Here's how the part is built. I have some questions about the finished solid (model axes, mm). A direction names the side the tool comes from. Round coordinates to 2 decimals unless told otherwise and drop trailing zeros. Order: outer loops, then holes, each group sorted by start corner. A loop starts at its lowest first (then second) coordinate and runs counter-clockwise, first axis right, second up. Notation, with made-up numbers: (-22.75, 37.5) -> (2.25, 37.5) arc R10 cw to (2.25, 53.5) -> close; hole circle Ø11 at (26.5, 42.25). An arc over 180 degrees is marked (long way). One line per item, written item: value.
```python
from build123d import *

# Parameters (mm, degrees)
SKICA1_W                 = 60
SKICA1_H                 = 100
P_IDAT_VYSUNUT_M1_DEPTH  = 30
SKICA2_W                 = 60
SKICA2_H                 = 30
P_IDAT_VYSUNUT_M2_DEPTH  = 80
SKICA3_R                 = 12.5
ODEBRAT_VYSUNUT_M1_DEPTH = 80
ZAOBLIT2_R               = 10
ZKOSEN_1_SIZE            = 5


with BuildPart() as part:
    # Skica1 → Přidat vysunutím1 (new body)
    with BuildSketch(Plane.XY):
        with Locations((30, 50)):
            Rectangle(SKICA1_W, SKICA1_H)
    extrude(amount=P_IDAT_VYSUNUT_M1_DEPTH)

    # Skica2 → Přidat vysunutím2 (add)
    with BuildSketch(Plane(origin=(0, 0, 0), x_dir=(-1, 0, 0), z_dir=(0, 0, -1))):
        with Locations((-30, 85)):
            Rectangle(SKICA2_W, SKICA2_H)
    extrude(amount=P_IDAT_VYSUNUT_M2_DEPTH)

    # Skica3 → Odebrat vysunutím1 (cut)
    with BuildSketch(Plane(origin=(0, 0, 0), x_dir=(-1, 0, 0), z_dir=(0, 0, -1))):
        with Locations((-30, 40)):
            Circle(SKICA3_R)
    extrude(amount=-ODEBRAT_VYSUNUT_M1_DEPTH, mode=Mode.SUBTRACT)

    # Zaoblit2
    zaoblit2_edges = [part.edges().sort_by_distance(p)[0] for p in [
        (30, 70, 0),
    ]]
    fillet(zaoblit2_edges, radius=ZAOBLIT2_R)

    # Zkosení1
    zkosen_1_edges = [part.edges().sort_by_distance(p)[0] for p in [
        (60, 0, 15),
        (0, 0, 15),
    ]]
    chamfer(zkosen_1_edges, length=ZKOSEN_1_SIZE)


solid = part.part
```
Q1. I need wall thicknesses on line 1 along Y through (x, z) = (30, 10.5); line 2 along Y through (x, z) = (7.5, -63.5); line 3 along Y through (x, z) = (34.5, 9). Which ranges of each line are inside material? Lowest first, please.
Answers:
line 1: 0 to 27.5, 52.5 to 100
line 2: 70 to 100
line 3: 0 to 28.34, 51.66 to 100
Q2. Which directions (+Z, -Z, +X, -X, +Y, -Y) give clear straight access to the entire face, cutting with the end or side of a thin tool? Please do faces 4 (the face through (30, 24, 0)), 5 (the face through (0, 73, -12)).
Answers:
face 4: -Z, +X, -X, -Y
face 5: +Z, -Z, -X, +Y, -Y
Q3. For P1, Ø1, axis at x = 52, z = -14.5, coming from the -Y side; P2, Ø1, axis at x = 30.5, y = 51, coming from the -Z side, each with a flat end and sliding along its axis, tell me the tip position at first contact or that it passes through.
Answers:
P1: y = 70
P2: through
Q4. If we mould it in two halves opening along X, with no side actions, what happens to faces 1 (the face through (23, 51, 30)), 2 (the face through (39.92, 32.394, 14.79)), 3 (the face through (2, 3, 15))? For each: pulls with the +X half, pulls with the -X half, needs draft (parallel to the pull), parting line crosses it, or undercut.
Answers:
face 1: needs draft
face 2: undercut
face 3: pulls with the -X half
Q5. I want a section at A-A on y = 40. Write out the boundary of the cut face in (x, z), then the cut area to 3 significant figures.
Answers:
outline: (0, 0) -> (17.5, 0) -> (17.5, 30) -> (0, 30) -> close; (42.5, 0) -> (60, 0) -> (60, 30) -> (42.5, 30) -> close
area: 1,050 mm2
Q6. I want a section at B-B on z = 21.5. Write out the boundary of the cut face in (x, y).
Answers:
outline: (0, 5) -> (5, 0) -> (55, 0) -> (60, 5) -> (60, 100) -> (0, 100) -> close; hole circle Ø25 at (30, 40)
Q7. I want a section at C-C on x = 30. Write out the boundary of the cut face in (y, z), then the cut area to 3 significant figures.
Answers:
outline: (0, 0) -> (27.5, 0) -> (27.5, 30) -> (0, 30) -> close; (52.5, 0) -> (60, 0) arc R10 cw to (70, -10) -> (70, -80) -> (100, -80) -> (100, 30) -> (52.5, 30) -> close
area: 4,670 mm2
Q8. I want a section at D-D on x = 48. Write out the boundary of the cut face in (y, z), then the cut area to 3 significant figures.
Answers:
outline: (0, 0) -> (60, 0) arc R10 cw to (70, -10) -> (70, -80) -> (100, -80) -> (100, 30) -> (0, 30) -> close
area: 5,420 mm2
